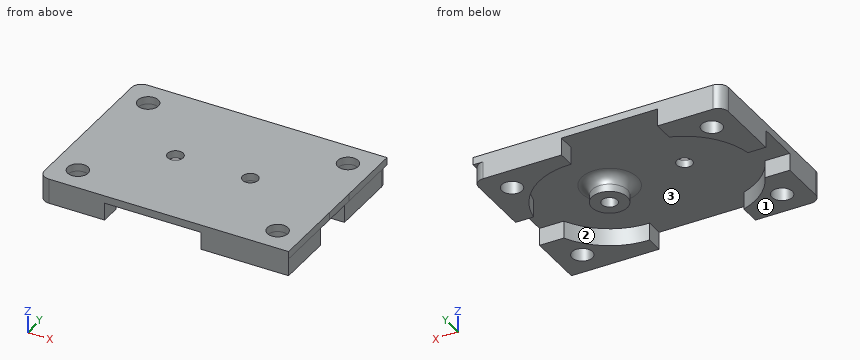
Autodesk Inventor part; units mm, degrees
ref_plane "YZ Plane" through (0, 0, 0) normal (1, 0, 0) x (0, 1, 0)
ref_plane "XZ Plane" through (0, 0, 0) normal (0, 1, 0) x (-1, 0, 0)
ref_plane "XY Plane" through (0, 0, 0) normal (0, 0, 1) x (1, 0, 0)
sketch "Skizze1" plane through (0, 0, 0) normal (0, 0, 1) x (1, 0, 0)
  line L0 (17.6969, -0.7673) -> (8.7277, -0.7347)
  arc A0 (8.2588, 6.1863) -> (8.7277, -0.7347) centre (0.2074, 2.1644) ccw
  line L1 (8.2588, 6.1863) -> (17.722, 6.1519)
  line L2 (17.7709, 19.6007) -> (17.722, 6.1519)
  line L3 (-32.2287, 19.7825) -> (17.7709, 19.6007)
  line L4 (-32.356, -15.2173) -> (-32.2287, 19.7825)
  line L5 (17.6436, -15.3991) -> (-32.356, -15.2173)
  line L6 (17.6969, -0.7673) -> (17.6436, -15.3991)
  circle A1 centre (-14.7925, 2.219) radius 1.45
  circle A2 centre (-14.7925, 2.219) radius 1.55
  circle A3 centre (0.2074, 2.1644) radius 1.55
  line L7 (17.6969, -0.7673) -> (17.722, 6.1519)
  circle A4 centre (-27.247, 14.7644) radius 2.05
  circle A5 centre (12.6619, -10.381) radius 2.05
  circle A6 centre (12.7528, 14.6189) radius 2.05
  circle A7 centre (-27.3379, -10.2355) radius 2.05
  point P0 (0, 0)
  dimension "d25" = 3.1
  dimension "d26" = 3.1
extrude "Extrusion1" add sketch "Skizze1" along normal blind 1.5 contours L6 L5 L4 L3 L2 L1 A0 L0 | L0 A0 L1 L7
sketch "Skizze6" plane through (0, 0, 0) normal (0, 0, -1) x (-1, 0, 0)
  circle A0 centre (14.7925, 2.219) radius 1.55
  circle A1 centre (-0.2074, 2.1644) radius 1.55
  circle A2 centre (-0.2074, 2.1644) radius 14.0891
  circle A3 centre (14.7925, 2.219) radius 14.0891
  line L0 (32.356, -15.2173) -> (-17.6436, -15.3991)
  line L1 (32.2287, 19.7825) -> (32.356, -15.2173)
  line L2 (-17.7709, 19.6007) -> (32.2287, 19.7825)
  line L3 (-17.6436, -15.3991) -> (-17.7709, 19.6007)
  line L4 (32.2287, 19.7825) -> (-17.7709, 19.6007)
  line L5 (32.356, -15.2173) -> (32.2287, 19.7825)
  line L6 (32.356, -15.2173) -> (-17.6436, -15.3991)
  circle A4 centre (27.3379, -10.2355) radius 2.05
  circle A5 centre (-12.7528, 14.6189) radius 2.05
  circle A6 centre (-12.6619, -10.381) radius 2.05
  circle A7 centre (27.247, 14.7644) radius 2.05
  circle A8 centre (-12.7528, 14.6189) radius 2.05
  circle A9 centre (27.247, 14.7644) radius 2.05
  circle A10 centre (27.3379, -10.2355) radius 2.05
  circle A11 centre (-12.6619, -10.381) radius 2.05
  point P0 (0, 0)
extrude "Extrusion7" add sketch "Skizze6" along normal blind 3.5
sketch "Skizze7" plane through (0, 0, -3.5) normal (0, 0, -1) x (-1, 0, 0)
  line L0 (-21.514, 4.474) -> (38.6582, 4.474)
  line L1 (38.6582, 4.474) -> (38.6582, -4.0646)
  line L2 (38.6582, -4.0646) -> (-21.514, -4.0646)
  line L3 (-21.514, -4.0646) -> (-21.514, 4.474)
  line L4 (-0.0651, 23.7233) -> (19.1842, 23.7233)
  line L5 (19.1842, 23.7233) -> (19.1842, -21.5163)
  line L6 (19.1842, -21.5163) -> (-0.0651, -21.5163)
  line L7 (-0.0651, -21.5163) -> (-0.0651, 23.7233)
  point P0 (0, 0)
extrude "Extrusion8" cut sketch "Skizze7" against normal up to surface (3.5 mm away)
sketch "Skizze2" plane through (0, 0, 0) normal (0, 0, -1) x (-1, 0, 0)
  circle A0 centre (-0.2074, 2.1644) radius 1.55
  arc A1 (-12.8448, -4.0646) -> (-0.0651, -11.924) centre (-0.2074, 2.1644) ccw
  circle A2 centre (-0.2074, 2.1644) radius 3.55
  point P0 (0, 0)
  dimension "d27" = 2
extrude "Extrusion2" add sketch "Skizze2" along normal blind 3.5
fillet "Rundung5" radius 2 4 edges at (3.7574, 2.1644, 0) (-32.356, -15.2173, -1) (17.7709, 19.6007, -1) (-32.2287, 19.7825, -1)
properties part number "GehäuseBack"
Design review of the part built by this model. Coordinates are the model's own, in mm. Face numbers are marked on the shaded views. Coordinates: 2 decimals unless noted, no trailing zeros. Order: outer loops, then holes, each group sorted by start corner. A loop starts at its lowest first (then second) coordinate and runs counter-clockwise, first axis right, second up. Notation, with made-up numbers: M -22.75,21 L 27.25,21 A21 cw 27.25,58 Z; hole C 50,-30.5 d5. An arc over 180 degrees is marked long. Answer as a JSON object with one key per item and string values. Group by question number.
1) For pin 1 (1 mm diameter, centred on y = 18, z = -2, fed in from -X); pin 2 (2 mm diameter, centred on y = 10.5, z = -1.5, fed in from +X); pin 3 (1 mm diameter, centred on x = -31, z = -1, fed in from +Y), all flat-tipped, find the tip position at first contact; note any pin that passes through.
2) Mouldability with a two-part tool opening along Y and no side actions: class the marked faces 1, 2 and 3 as pulls with the +Y half, pulls with the -Y half, needs draft (parallel to the pull), parting line crosses it, or undercut.
3) Wall thickness on L1, parallel to X at y = -12.5, z = -1.65; L2, parallel to Y at x = 11, z = -2.85; L3, parallel to X at y = 13, z = -1: over which ranges is each line inside the solid? List them lowest first.
4) Add section A-A, the plane z = -2.85. Count the separate pieces of the cut face and the enclosed holes in it, then the cut area to 3 significant figures.
5) Add section B-B, the plane x = -28. Write out the cut boundary in (y, z).
6) Add section C-C, the plane x = -20.5. Write out the cut boundary in (y, z), then the cut area to 3 significant figures.
Computed values:
{
 "1": {"pin 1": "stops at x = -32.24", "pin 2": "stops at x = 17.74", "pin 3": "stops at y = 19.76"},
 "2": {"face 1": "needs draft", "face 2": "undercut", "face 3": "undercut"},
 "3": {"L1": "x = -32.35 to -19.18, 0.07 to 17.65", "L2": "y = -15.37 to -11.58, -9.18 to -6.89, 11.22 to 13.56, 15.68 to 19.63", "L3": "x = -32.25 to -28.29, -26.2 to -23.86, 9.21 to 11.5, 14.01 to 17.75"},
 "4": {"separate pieces": "5", "enclosed holes": "5", "area": "483 mm^2"},
 "5": {"outline": "M -15.23,-3.5 L -12.18,-3.5 L -12.18,1.5 L -15.23,1.5 Z; M -8.3,-3.5 L -4.06,-3.5 L -4.06,0 L 7.12,0 L 7.12,-3.5 L 12.86,-3.5 L 12.86,1.5 L -8.3,1.5 Z; M 16.67,-3.5 L 19.77,-3.5 L 19.77,1.5 L 16.67,1.5 Z"},
 "6": {"outline": "M -15.26,-3.5 L -10.66,-3.5 L -10.66,0 L 15.1,0 L 15.1,-3.5 L 19.74,-3.5 L 19.74,1.5 L -15.26,1.5 Z", "area": "84.8 mm^2"}
}
